from build123d import *

# Parameters (mm, degrees)
F0_W     = 152.4
F0_H     = 644.906
F0_R     = 43.053
F1_DEPTH = 177.8
F3_D     = 10.16
F3_DEPTH = 50.8
F3_TIP   = 3.0523719447
F5_DEPTH = 101.6
F8_DEPTH = 38.1
F9_D     = 6.35
F9_DEPTH = 38.1
F9_TIP   = 1.9077324654
F10_R    = 6.35


# Not quite as in the source:
# - a feature names something its author has since deleted; it is built from what else it names


with BuildPart() as f1:
    # F0 (on Top) → F1 (new body)
    with BuildSketch(Plane.XY):
        with Locations((0, 22.9516405373)):
            Rectangle(F0_W, F0_H)
        with Locations((0, -231.0483594627)):
            Circle(F0_R, mode=Mode.SUBTRACT)
        with Locations((0, -129.4483594627)):
            Circle(F0_R, mode=Mode.SUBTRACT)
        with Locations((0, -27.8483594627)):
            Circle(F0_R, mode=Mode.SUBTRACT)
        with Locations((0, 73.7516405373)):
            Circle(F0_R, mode=Mode.SUBTRACT)
        with Locations((0, 175.3516405373)):
            Circle(F0_R, mode=Mode.SUBTRACT)
        with Locations((0, 276.9516405373)):
            Circle(F0_R, mode=Mode.SUBTRACT)
    extrude(amount=F1_DEPTH)

    # F3
    with Locations(Plane.XY.offset(177.8)):
        with Locations((-60.96, -284.2613594627), (60.96, -284.2613594627), (-60.96, -180.2483594627), (60.96, -180.2483594627), (-60.96, -78.6483594627), (60.96, -78.6483594627), (-60.96, 22.9516405373), (60.96, 22.9516405373), (-60.96, 124.5516405373), (60.96, 124.5516405373), (-60.96, 226.1516405373), (60.96, 226.1516405373), (-60.96, 330.1646405373), (60.96, 330.1646405373)):
            Hole(F3_D / 2, depth=F3_DEPTH)
            with Locations((0, 0, -(F3_DEPTH + F3_TIP / 2))):  # 118° drill point
                Cone(0, F3_D / 2, F3_TIP, mode=Mode.SUBTRACT)

    # F4 (on face) → F5 (cut)
    with BuildSketch(Plane.XY.offset(177.8)):
        with BuildLine():
            ThreePointArc((-39.5301250083, -173.9482047983), (-41.9112858201, -174.185525814), (-43.0385000083, -176.2963636216))
            Line((-43.0385000083, -176.2963636216), (-43.0385000083, -184.2003553039))
            ThreePointArc((-43.0385000083, -184.2003553039), (-41.9112858201, -186.3111931115), (-39.5301250083, -186.5485141272))
            Line((-39.5301250083, -186.5485141272), (-29.947149504, -182.596518286))
            ThreePointArc((-29.947149504, -182.596518286), (-28.375524504, -180.2483594627), (-29.947149504, -177.9002006395))
            Line((-29.947149504, -177.9002006395), (-39.5301250083, -173.9482047983))
        make_face()
        with BuildLine():
            Line((42.8050714591, -184.1785549312), (42.7631932188, -176.2809378323))
            ThreePointArc((42.7631932188, -176.2809378323), (41.6287769855, -174.1787422376), (39.2512218362, -173.9477486864))
            Line((39.2512218362, -173.9477486864), (29.7178532592, -177.8965572358))
            ThreePointArc((29.7178532592, -177.8965572358), (28.149861111, -180.2451799461), (29.7214853508, -182.5913737277))
            Line((29.7214853508, -182.5913737277), (39.2967321682, -186.5401822772))
            ThreePointArc((39.2967321682, -186.5401822772), (41.6834844647, -186.299108133), (42.8050714591, -184.1785549312))
        make_face()
        with BuildLine():
            ThreePointArc((-39.5301250083, -72.3482047983), (-41.9112858201, -72.585525814), (-43.0385000083, -74.6963636216))
            Line((-43.0385000083, -74.6963636216), (-43.0385000083, -82.6003553039))
            ThreePointArc((-43.0385000083, -82.6003553039), (-41.9112858201, -84.7111931115), (-39.5301250083, -84.9485141272))
            Line((-39.5301250083, -84.9485141272), (-29.947149504, -80.996518286))
            ThreePointArc((-29.947149504, -80.996518286), (-28.375524504, -78.6483594627), (-29.947149504, -76.3002006395))
            Line((-29.947149504, -76.3002006395), (-39.5301250083, -72.3482047983))
        make_face()
        with BuildLine():
            Line((42.2662900285, -82.5723412323), (42.2244772598, -74.6870711239))
            ThreePointArc((42.2244772598, -74.6870711239), (41.0880034509, -72.579426147), (38.7049289993, -72.3455539051))
            Line((38.7049289993, -72.3455539051), (29.1514032422, -76.2881889593))
            ThreePointArc((29.1514032422, -76.2881889593), (27.5756070282, -78.6451741517), (29.1550254915, -80.9997336057))
            Line((29.1550254915, -80.9997336057), (38.7503640173, -84.9423686599))
            ThreePointArc((38.7503640173, -84.9423686599), (41.1426684979, -84.6983979341), (42.2662900285, -82.5723412323))
        make_face()
        with BuildLine():
            ThreePointArc((-39.5301250083, 29.2517952017), (-41.9112858201, 29.014474186), (-43.0385000083, 26.9036363784))
            Line((-43.0385000083, 26.9036363784), (-43.0385000083, 18.9996446961))
            ThreePointArc((-43.0385000083, 18.9996446961), (-41.9112858201, 16.8888068885), (-39.5301250083, 16.6514858728))
            Line((-39.5301250083, 16.6514858728), (-29.947149504, 20.603481714))
            ThreePointArc((-29.947149504, 20.603481714), (-28.375524504, 22.9516405373), (-29.947149504, 25.2997993605))
            Line((-29.947149504, 25.2997993605), (-39.5301250083, 29.2517952017))
        make_face()
        with BuildLine():
            Line((41.7277221449, 18.9936006532), (41.6855505867, 26.946533154))
            ThreePointArc((41.6855505867, 26.946533154), (40.5605129606, 29.0230527195), (38.2087640486, 29.2396634781))
            Line((38.2087640486, 29.2396634781), (28.7869515979, 25.2631972277))
            ThreePointArc((28.7869515979, 25.2631972277), (27.2569622126, 22.9547929732), (28.7906370523, 20.6488356434))
            Line((28.7906370523, 20.6488356434), (38.2546210612, 16.672369393))
            ThreePointArc((38.2546210612, 16.672369393), (40.6154092138, 16.8989805748), (41.7277221449, 18.9936006532))
        make_face()
        with BuildLine():
            ThreePointArc((-39.2389715781, 130.8516052404), (-41.6215382557, 130.6118153154), (-42.7459306424, 128.4976098044))
            Line((-42.7459306424, 128.4976098044), (-42.7295716504, 120.5911560789))
            ThreePointArc((-42.7295716504, 120.5911560789), (-41.6001784129, 118.4841132501), (-39.2212020873, 118.2482526776))
            Line((-39.2212020873, 118.2482526776), (-29.635241547, 122.2014795403))
            ThreePointArc((-29.635241547, 122.2014795403), (-28.0636166616, 124.5504011364), (-29.6366520458, 126.8983783776))
            Line((-29.6366520458, 126.8983783776), (-39.2389715781, 130.8516052404))
        make_face()
        with BuildLine():
            Line((41.1269060209, 120.5623967021), (41.1269060209, 128.5408843724))
            ThreePointArc((41.1269060209, 128.5408843724), (40.0124074762, 130.6155991372), (37.6672454799, 130.8318480041))
            Line((37.6672454799, 130.8318480041), (28.2579874063, 126.8426041689))
            ThreePointArc((28.2579874063, 126.8426041689), (26.740926903, 124.5516405373), (28.2579874063, 122.2606769056))
            Line((28.2579874063, 122.2606769056), (37.6672454799, 118.2714330704))
            ThreePointArc((37.6672454799, 118.2714330704), (40.0124074762, 118.4876819373), (41.1269060209, 120.5623967021))
        make_face()
        with BuildLine():
            Line((-39.4786105583, 219.9656601087), (-29.866499751, 224.1805924273))
            ThreePointArc((-29.866499751, 224.1805924273), (-28.4228668084, 226.3396283374), (-29.8678000125, 228.4977942646))
            Line((-29.8678000125, 228.4977942646), (-39.5349560025, 232.4619589189))
            ThreePointArc((-39.5349560025, 232.4619589189), (-41.9134370658, 232.2213103618), (-43.0385000083, 230.1119698791))
            Line((-43.0385000083, 230.1119698791), (-43.0385000083, 222.2917467873))
            ThreePointArc((-43.0385000083, 222.2917467873), (-41.8879192273, 220.1655123145), (-39.4786105583, 219.9656601087))
        make_face()
        with BuildLine():
            Line((40.650672554, 222.1092328525), (40.6076142213, 230.2293979276))
            ThreePointArc((40.6076142213, 230.2293979276), (39.515765156, 232.1937343917), (37.2723493523, 232.3272920851))
            Line((37.2723493523, 232.3272920851), (28.7048957748, 228.2672095476))
            ThreePointArc((28.7048957748, 228.2672095476), (27.3697030623, 226.15467094), (28.7089851923, 224.0447225226))
            Line((28.7089851923, 224.0447225226), (37.3194971026, 219.9846399851))
            ThreePointArc((37.3194971026, 219.9846399851), (39.5711951198, 220.1279668388), (40.650672554, 222.1092328525))
        make_face()
    extrude(amount=-F5_DEPTH, mode=Mode.SUBTRACT)

    # F7 (on face) → F8 (join)
    with BuildSketch(Plane(origin=(0, 0, 0), x_dir=(1, 0, 0), z_dir=(0, 0, -1))):
        Polygon((76.2, -345.4046405373), (76.2, 299.4986176491), (76.2, 299.5013594627), (-76.2, 299.5013594627), (-76.2, -345.4046405373), align=None)
        Polygon((-60.96, -321.8358690433), (-60.96, 286.0599543583), (60.96, 286.0599543583), (60.96, -331.9680405373), (-60.96, -331.9680405373), align=None, mode=Mode.SUBTRACT)
    extrude(amount=F8_DEPTH)

    # F9 (one way)
    with BuildSketch(Plane.XY):
        with Locations((-68.58, -78.6483594627), (68.58, -78.6483594627)):
            Circle(F9_D / 2)
    extrude(amount=-F9_DEPTH, mode=Mode.SUBTRACT)
    with Locations(Plane.XY):
        with Locations((-68.58, -78.6483594627), (68.58, -78.6483594627)):
            with Locations((0, 0, -(F9_DEPTH + F9_TIP / 2))):  # 118° drill point
                Cone(0, F9_D / 2, F9_TIP, mode=Mode.SUBTRACT)

    # F10
    f10_edges = [f1.edges().sort_by_distance(p)[0] for p in [
        (60.96, -286.059954, -19.05),
        (-60.96, -286.059954, -19.05),
        (60.96, 331.968041, -19.05),
        (-60.96, 331.968041, -19.05),
    ]]
    fillet(f10_edges, radius=F10_R)


solid = f1.part
The listing builds one solid part. Answer for the finished solid, in the listing's coordinates (mm). A direction names the side the tool comes from. Give positions to 0.01 mm unless a question says otherwise; leave off trailing zeros. Write each loop counter-clockwise with the first axis right and the second up, starting at its lowest first coordinate (ties: lowest second). Pieces come first, ordered by that corner, then holes.
1) Section C-C (z = 29) is taken. Write down the section's boundary in (x, y).
2) Section A-A (y = -108) is taken. Write down the section's boundary in (x, z).
3) For a pull along X with two mould halves and no side action, classify faces 1 (the face through (-76.2, 18, 71)), 2 (the face through (76.2, 27, 71)), 3 (the face through (-60.96, 27, -19)) as pulls with the +X half, pulls with the -X half, needs draft (parallel to the pull), parting line crosses it, or undercut.
4) Section D-D (y = 148.5) is taken. Write down the section's boundary in (x, z).
5) A tool of negligible diameter and unlimited length cuts with its end or side. For faces 4 (the face through (-43.01, -25.96, 87.66)), 5 (the face through (60.96, 19, -19)), 6 (the face through (37, -180, 76.2)), from which of +Z, -Z, +X, -X, +Y, -Y can it reach the whole face along a straight path? Write none if from no direction.
6) Given P1, Ø3, axis at x = -21, y = -167.5, coming from the -Z side; P2, Ø4, axis at x = 37, y = -182.5, coming from the +Z side, each flat-ended and moving along its own axis, determine where each tip first touches the part or whether it passes through.
7) Find the intervals of material crossed by L1, parallel to Y at x = -39, z = -21.5; L2, parallel to X at y = 176, z = 56; L3, parallel to X at y = 27, z = 100, in increasing order.
8) Section B-B (x = 0) is taken. Count the separate pieces of the cut face and the enclosed holes in it, and give its area (3 significant figures).
Response:
1. outline: (-76.2, -299.5) - (76.2, -299.5) - (76.2, 345.4) - (-76.2, 345.4) - close; hole circle Ø86.11 at (0, -231.05); hole circle Ø86.11 at (0, -129.45); hole circle Ø86.11 at (0, -27.85); hole circle Ø86.11 at (0, 73.75); hole circle Ø86.11 at (0, 175.35); hole circle Ø86.11 at (0, 276.95)
2. outline: (-76.2, -38.1) - (-60.96, -38.1) - (-60.96, 0) - (-37.33, 0) - (-37.33, 177.8) - (-76.2, 177.8) - close; (37.33, 0) - (60.96, 0) - (60.96, -38.1) - (76.2, -38.1) - (76.2, 177.8) - (37.33, 177.8) - close
3. face 1: pulls with the -X half
3. face 2: pulls with the +X half
3. face 3: undercut
4. outline: (-76.2, -38.1) - (-60.96, -38.1) - (-60.96, 0) - (-33.65, 0) - (-33.65, 177.8) - (-76.2, 177.8) - close; (33.65, 0) - (60.96, 0) - (60.96, -38.1) - (76.2, -38.1) - (76.2, 177.8) - (33.65, 177.8) - close
5. face 4: +Z, -Z
5. face 5: -Z
5. face 6: +Z
6. P1: stops at z = 0
6. P2: stops at z = 76.2
7. L1: y = -299.5 to -286.06, 331.97 to 345.4
7. L2: x = -76.2 to -43.05, 43.05 to 76.2
7. L3: x = -76.2 to -43.04, -34.07 to 32.9, 41.68 to 76.2
8. separate pieces: 7
8. enclosed holes: 0
8. area: 23,800 mm2
